Work out the finished part from the listing and answer in its coordinate system (mm). A direction names the side the tool comes from. Round coordinates to 2 decimals unless told otherwise and drop trailing zeros. Write each loop counter-clockwise with the first axis right and the second up, starting at its lowest first coordinate (ties: lowest second). Pieces come first, ordered by that corner, then holes. Notation, with made-up numbers: (20, 49) - (35, 49) arc R21 cw to (35, 88) - close; hole circle Ø8 at (42.5, 17). An arc over 180 degrees is marked (long way). Answer as a JSON object with one key per item and string values.
```python
from build123d import *

# Parameters (mm, degrees)
SKETCH1_W           = 6
SKETCH1_H           = 4
BOSS_EXTRUDE1_DEPTH = 1.25
BOSS_EXTRUDE2_DEPTH = 1.5
BOSS_EXTRUDE3_START = 1.5
BOSS_EXTRUDE3_DEPTH = 1.5


with BuildPart() as part:
    # Sketch1 → Boss-Extrude1 (new body)
    with BuildSketch(Plane.XY):
        Rectangle(SKETCH1_W, SKETCH1_H)
    extrude(amount=-BOSS_EXTRUDE1_DEPTH)

    # Sketch1<3> → Boss-Extrude2 (add)
    with BuildSketch(Plane.XY):
        Polygon((0.5, 2), (-3, 1), (-3, -2), (3, -2), (3, 1), align=None)
    extrude(amount=BOSS_EXTRUDE2_DEPTH)

    # Sketch1<4> → Boss-Extrude3 (add)
    with BuildSketch(Plane.XY.offset(BOSS_EXTRUDE3_START)):
        Polygon((-3, 2), (-3, 1), (0.5, 2), align=None)
        Polygon((0.5, 2), (-3, 1), (-3, -2), (3, -2), (3, 1), align=None)
        Polygon((3, 2), (0.5, 2), (3, 1), align=None)
    extrude(amount=BOSS_EXTRUDE3_DEPTH)


solid = part.part
```
Item 1: For faces 1 (the flat face through (1.77, 1.49, 0.74)), 2 (the flat face through (-1.226, 1.507, 0.74)), 3 (the flat face through (-3, 0, 1)), determine the directions among +Z, -Z, +X, -X, +Y, -Y from which every point of the face is accessible in a straight line to the end or side of a thin tool.
Results found:
{"face 1": "+X, +Y", "face 2": "-X, +Y", "face 3": "+Z, -Z, -X, +Y, -Y"}
Item 2: A cutting plane is placed at B-B (y = 1.1). Write down the section's boundary in (x, z).
Results found:
{"outline": "(-3, -1.25) - (3, -1.25) - (3, 0) - (2.75, 0) - (2.75, 1.5) - (3, 1.5) - (3, 3) - (-3, 3) - (-3, 1.5) - (-2.65, 1.5) - (-2.65, 0) - (-3, 0) - close"}
Item 3: A cutting plane is placed at A-A (x = 1.05). Write down the section's boundary in (y, z), and give its area (3 significant figures).
Results found:
{"outline": "(-2, -1.25) - (2, -1.25) - (2, 0) - (1.78, 0) - (1.78, 1.5) - (2, 1.5) - (2, 3) - (-2, 3) - close", "area": "16.7 mm²"}
Item 4: A cutting plane is placed at D-D (x = 2.05). Write down the section's boundary in (y, z).
Results found:
{"outline": "(-2, -1.25) - (2, -1.25) - (2, 0) - (1.38, 0) - (1.38, 1.5) - (2, 1.5) - (2, 3) - (-2, 3) - close"}
Item 5: Determine the mould class of faces 4 (the flat face through (2.3, 1.7, 0)), 5 (the flat face through (2.3, 1.7, 1.5)), 6 (the flat face through (0, 0, 3)), 7 (the flat face through (0, 2, -1)) for opening direction Z: pulls with the +Z half, pulls with the -Z half, needs draft (parallel to the pull), parting line crosses it, or undercut.
Results found:
{"face 4": "undercut", "face 5": "undercut", "face 6": "pulls with the +Z half", "face 7": "needs draft"}
Item 6: A cutting plane is placed at C-C (z = 0.3). Write down the section's boundary in (x, y).
Results found:
{"outline": "(-3, -2) - (3, -2) - (3, 1) - (0.5, 2) - (-3, 1) - close"}
Item 7: Consider line 1 along Z through (x, y) = (2.75, 1.15); line 2 along Y through (x, z) = (-2.45, 0.7); line 3 along Y through (x, z) = (-1.9, 0.1). Determine where each line is inside the solid, lowest interval first.
Results found:
{"line 1": "-1.25 to 0, 1.5 to 3", "line 2": "-2 to 1.16", "line 3": "-2 to 1.31"}
